Geometry: final body of the model. Coordinates: model frame, mm. Give positions to 0.01 mm unless a question says otherwise; leave off trailing zeros. Loops run counter-clockwise (first coordinate to the right, second up) from the corner with the lowest first, then second, coordinate; pieces in that order, holes last. Notation, with made-up numbers: (39, -31) -> (62, -31) arc R25 ccw to (62, 3) -> close; hole circle Ø1 at (60, 53.5). An arc over 180 degrees is marked (long way). Answer in a Markdown table with one row per item. Add a question column.
1) Section query C-C (y = 96.5). Return the cut outline in (x, z), plus the area to 3 significant figures.
2) First-contact query: P1, Ø2, axis at x = 0, y = 68.03, coming from the -Z side; P2, Ø1.3, axis at y = 115.5, z = -8, coming from the +X side; P3, Ø2, axis at x = -1, y = 112, coming from the +Z side. Flat tips, straight axial feed; report the tip coordinate or a pass-through.
3) Section query A-A (z = 0). Return the cut outline in (x, y) (1 decimal), plus the area to 3 significant figures.
4) Section query B-B (x = -3.75). Return the cut outline in (y, z) (1 decimal), plus the area to 3 significant figures.
5) Line query: line 1 (Z direction, x = 3.3, y = 115.11); line 2 (Y direction, x = -1.75, z = 16); line 3 (Z direction, x = 4.25, y = 46) (3 decimals). Output: solid intervals per line, ascending. Write a range as from..to.
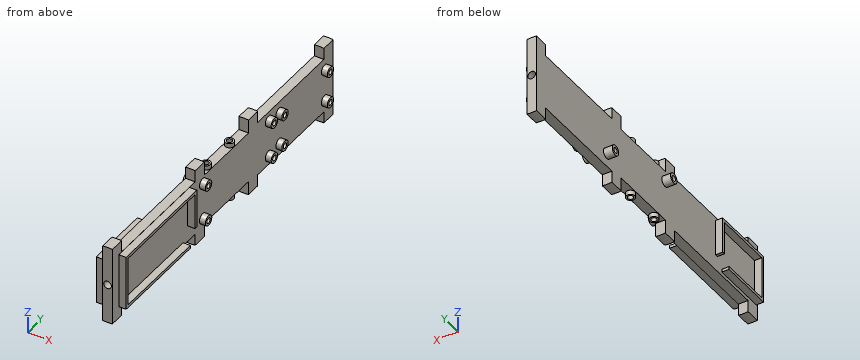
```python
from build123d import *

# Parameters (mm, degrees)
SKETCH1_R                            = 1.651
BOSS_EXTRUDE1_DEPTH                  = 152.4
SKETCH2_W                            = 4.191
SKETCH2_H                            = 30.48
CUT_EXTRUDE1_DEPTH                   = 6.096
SKETCH3_R                            = 1.905
BOSS_EXTRUDE2_DEPTH                  = 1.905
SKETCH4_R                            = 1.17475
CUT_EXTRUDE2_DEPTH                   = 6.35
SKETCH7_R                            = 2.2225
SKETCH7_R_2                          = 1.1811
STRATOLOGGER_MOUNTS_DEPTH            = 2.54
SKETCH8_R                            = 2.2225
SKETCH8_R_2                          = 1.1811
EASYMINI_MOUNTS_DEPTH                = 2.54
SKETCH9_W                            = 7.62
SKETCH9_H                            = 50.8
SKETCH9_H_2                          = 45.72
WIRE_PASSTHROUGHS_DEPTH              = 154.425737584
SKETCH12_R                           = 2.2225
SKETCH12_R_2                         = 1.1811
EGGFINDER_MINI_MOUNTS_SMALL_2S_DEPTH = 3.81
F_1S_LIPO_MOUINTS_SMALL_2S_DEPTH     = 3.175
BOSS_EXTRUDE5_DEPTH                  = 3.175


with BuildPart() as part:
    # Sketch1 → Boss-Extrude1 (new body)
    with BuildSketch(Plane(origin=(0, 0, 0), x_dir=(1, 0, 0), z_dir=(0, 1, 0))):
        with BuildLine():
            Line((2.0955, -17.080437699), (2.0955, 17.080437699))
            ThreePointArc((2.0955, 17.080437699), (0, 17.2085), (-2.0955, 17.080437699))
            Line((-2.0955, 17.080437699), (-2.0955, -17.080437699))
            ThreePointArc((-2.0955, -17.080437699), (0, -17.2085), (2.0955, -17.080437699))
        make_face()
        with Locations(Location((0, 0, 0), (0, 0, 90))):
            Circle(SKETCH1_R, mode=Mode.SUBTRACT)
    extrude(amount=BOSS_EXTRUDE1_DEPTH)

    # Sketch2 → Cut-Extrude1 (cut)
    with BuildSketch(Plane(origin=(0, 0, -17.2085), x_dir=(-1, 0, 0), z_dir=(0, 0, -1))):
        with Locations((0, 78.74)):
            Rectangle(SKETCH2_W, SKETCH2_H)
    cut_extrude1 = extrude(amount=-CUT_EXTRUDE1_DEPTH, mode=Mode.SUBTRACT)

    # Sketch3 → Boss-Extrude2 (add)
    with BuildSketch(Plane(origin=(0, 0, -11.1125), x_dir=(-1, 0, 0), z_dir=(0, 0, -1))):
        with Locations(Location((0, 68.0339, 0), (0, 0, 180))):
            Circle(SKETCH3_R)
        with Locations(Location((0, 84.1629, 0), (0, 0, 180))):
            Circle(SKETCH3_R)
    boss_extrude2 = extrude(amount=BOSS_EXTRUDE2_DEPTH)

    # Sketch4 → Cut-Extrude2 (cut)
    with BuildSketch(Plane(origin=(0, 0, -13.0175), x_dir=(-1, 0, 0), z_dir=(0, 0, -1))):
        with Locations((0, 84.1629)):
            Circle(SKETCH4_R)
        with Locations((0, 68.0339)):
            Circle(SKETCH4_R)
    cut_extrude2 = extrude(amount=-CUT_EXTRUDE2_DEPTH, mode=Mode.SUBTRACT)

    # Mirror1: Cut-Extrude1, Boss-Extrude2, Cut-Extrude2 across plane
    add(cut_extrude1.mirror(Plane.XY), mode=Mode.SUBTRACT)
    add(boss_extrude2.mirror(Plane.XY))
    add(cut_extrude2.mirror(Plane.XY), mode=Mode.SUBTRACT)

    # Sketch7 → Stratologger Mounts (add)
    # profile 1 of 4: a face of its own
    with BuildSketch(Plane(origin=(2.0955, 0, 0), x_dir=(0, 0, -1), z_dir=(1, 0, 0))):
        with Locations(Location((8.001, 62.357, 0), (0, 0, 180))):
            Circle(SKETCH7_R)
        with Locations((8.001, 62.357)):
            Circle(SKETCH7_R_2, mode=Mode.SUBTRACT)
    # profile 2 of 4: a face of its own
    with BuildSketch(Plane(origin=(2.0955, 0, 0), x_dir=(0, 0, -1), z_dir=(1, 0, 0))):
        with Locations(Location((-8.001, 62.357, 0), (0, 0, 180))):
            Circle(SKETCH7_R)
        with Locations((-8.001, 62.357)):
            Circle(SKETCH7_R_2, mode=Mode.SUBTRACT)
    # profile 3 of 4: a face of its own
    with BuildSketch(Plane(origin=(2.0955, 0, 0), x_dir=(0, 0, -1), z_dir=(1, 0, 0))):
        with Locations(Location((-8.001, 107.823, 0), (0, 0, 180))):
            Circle(SKETCH7_R)
        with Locations((-8.001, 107.823)):
            Circle(SKETCH7_R_2, mode=Mode.SUBTRACT)
    # profile 4 of 4: a face of its own
    with BuildSketch(Plane(origin=(2.0955, 0, 0), x_dir=(0, 0, -1), z_dir=(1, 0, 0))):
        with Locations(Location((8.001, 107.823, 0), (0, 0, 180))):
            Circle(SKETCH7_R)
        with Locations((8.001, 107.823)):
            Circle(SKETCH7_R_2, mode=Mode.SUBTRACT)
    extrude(amount=STRATOLOGGER_MOUNTS_DEPTH)

    # Sketch8 → EasyMini Mounts (add)
    # profile 1 of 4: a face of its own
    with BuildSketch(Plane(origin=(2.0955, 0, 0), x_dir=(0, 0, -1), z_dir=(1, 0, 0))):
        with Locations(Location((7, 115.11, 0), (0, 0, 180))):
            Circle(SKETCH8_R)
        with Locations((7, 115.11)):
            Circle(SKETCH8_R_2, mode=Mode.SUBTRACT)
    # profile 2 of 4: a face of its own
    with BuildSketch(Plane(origin=(2.0955, 0, 0), x_dir=(0, 0, -1), z_dir=(1, 0, 0))):
        with Locations(Location((-7, 115.11, 0), (0, 0, 180))):
            Circle(SKETCH8_R)
        with Locations((-7, 115.11)):
            Circle(SKETCH8_R_2, mode=Mode.SUBTRACT)
    # profile 3 of 4: a face of its own
    with BuildSketch(Plane(origin=(2.0955, 0, 0), x_dir=(0, 0, -1), z_dir=(1, 0, 0))):
        with Locations(Location((-7, 146.51, 0), (0, 0, 180))):
            Circle(SKETCH8_R)
        with Locations((-7, 146.51)):
            Circle(SKETCH8_R_2, mode=Mode.SUBTRACT)
    # profile 4 of 4: a face of its own
    with BuildSketch(Plane(origin=(2.0955, 0, 0), x_dir=(0, 0, -1), z_dir=(1, 0, 0))):
        with Locations(Location((7, 146.51, 0), (0, 0, 180))):
            Circle(SKETCH8_R)
        with Locations((7, 146.51)):
            Circle(SKETCH8_R_2, mode=Mode.SUBTRACT)
    extrude(amount=EASYMINI_MOUNTS_DEPTH)

    # Sketch9 → Wire Passthroughs (cut, through all)
    with BuildSketch(Plane(origin=(2.0955, 0, 0), x_dir=(0, 0, -1), z_dir=(1, 0, 0))):
        with Locations((15.810437699, 31.75)):
            Rectangle(SKETCH9_W, SKETCH9_H)
        with Locations((-15.810437699, 31.75)):
            Rectangle(SKETCH9_W, SKETCH9_H)
        with Locations((-15.810437699, 123.19)):
            Rectangle(SKETCH9_W, SKETCH9_H_2)
        with Locations((15.810437699, 123.19)):
            Rectangle(SKETCH9_W, SKETCH9_H_2)
    extrude(amount=-WIRE_PASSTHROUGHS_DEPTH, mode=Mode.SUBTRACT)

    # Sketch12 → Eggfinder Mini Mounts Small 2s (add)
    # profile 1 of 2: a face of its own
    with BuildSketch(Plane.ZY.offset(2.0955)):
        with Locations(Location((-6.2865, 103.9495, 0), (0, 0, 180))):
            Circle(SKETCH12_R)
        with Locations((-6.2865, 103.9495)):
            Circle(SKETCH12_R_2, mode=Mode.SUBTRACT)
    # profile 2 of 2: a face of its own
    with BuildSketch(Plane.ZY.offset(2.0955)):
        with Locations(Location((6.2865, 63.6905, 0), (0, 0, 180))):
            Circle(SKETCH12_R)
        with Locations((6.2865, 63.6905)):
            Circle(SKETCH12_R_2, mode=Mode.SUBTRACT)
    extrude(amount=EGGFINDER_MINI_MOUNTS_SMALL_2S_DEPTH)

    # Sketch13 → 1s LiPo Mouints Small 2s (add)
    with BuildSketch(Plane.ZY.offset(2.0955)):
        Polygon((-9.134134948, 1.905), (9.134134948, 1.905), (9.134134948, 27.675), (-5.324134948, 27.675), (-5.324134948, 28.945), (10.404134948, 28.945), (10.404134948, 0.635), (-10.404134948, 0.635), (-10.404134948, 24.5), (-9.134134948, 24.5), align=None)
    extrude(amount=F_1S_LIPO_MOUINTS_SMALL_2S_DEPTH)

    # Sketch14 → Boss-Extrude5 (add)
    with BuildSketch(Plane(origin=(2.0955, 0, 0), x_dir=(0, 0, -1), z_dir=(1, 0, 0))):
        Polygon((-10.635, 5.715), (10.635, 5.715), (10.635, 48.81), (11.905, 48.81), (11.905, 4.445), (-11.905, 4.445), (-11.905, 53.255), (4.92, 53.255), (4.92, 51.985), (-10.635, 51.985), align=None)
    extrude(amount=BOSS_EXTRUDE5_DEPTH)


solid = part.part
```
Evaluation:
| question | item | result |
|---|---|---|
| 1 | outline | (-2.1, -17.08) arc R17.21 ccw to (2.1, -17.08) -> (2.1, 17.08) arc R17.21 ccw to (-2.1, 17.08) -> close; hole circle Ø3.3 at (0, 0) |
| 1 | area | 135 mm² |
| 2 | P1 | z = -6.67 |
| 2 | P2 | x = 4.64 |
| 2 | P3 | z = 12 |
| 3 | outline | (-5.3, 0.6) -> (-2.1, 0.6) -> (-2.1, 0) -> (-1.7, 0) -> (-1.7, 152.4) -> (-2.1, 152.4) -> (-2.1, 28.9) -> (-5.3, 28.9) -> (-5.3, 27.7) -> (-2.1, 27.7) -> (-2.1, 1.9) -> (-5.3, 1.9) -> close; (1.7, 0) -> (2.1, 0) -> (2.1, 4.4) -> (5.3, 4.4) -> (5.3, 5.7) -> (2.1, 5.7) -> (2.1, 52) -> (5.3, 52) -> (5.3, 53.3) -> (2.1, 53.3) -> (2.1, 152.4) -> (1.7, 152.4) -> close |
| 3 | area | 152 mm² |
| 4 | outline | (0.6, -10.4) -> (24.5, -10.4) -> (24.5, -9.1) -> (1.9, -9.1) -> (1.9, 9.1) -> (27.7, 9.1) -> (27.7, -5.3) -> (28.9, -5.3) -> (28.9, 10.4) -> (0.6, 10.4) -> close; circle Ø4.4 at (63.7, 6.3); circle Ø4.4 at (103.9, -6.3); hole circle Ø2.4 at (63.7, 6.3); hole circle Ø2.4 at (103.9, -6.3) |
| 4 | area | 130 mm² |
| 5 | line 1 | -9.22..-8.18, -5.82..-4.78, 4.78..5.82, 8.18..9.22 |
| 5 | line 2 | 0..6.35, 57.15..63.5, 93.98..100.33, 146.05..152.4 |
| 5 | line 3 | -11.905..-10.635, 10.635..11.905 |
